Design review of the part shown in the three views and the two pictorial views. Dimensions are in mm from the part's minimum x, y and z. Round coordinates to 2 decimals unless told otherwise and drop trailing zeros. Write each loop counter-clockwise with the first axis right and the second up, starting at its lowest first coordinate (ties: lowest second). Pieces come first, ordered by that corner, then holes. Notation, with made-up numbers: (26.5, 32) - (56.5, 32) arc R30 ccw to (56.5, 71) - close; hole circle Ø1 at (18, 4.5). An arc over 180 degrees is marked (long way). Use one line per item in the form item = value.
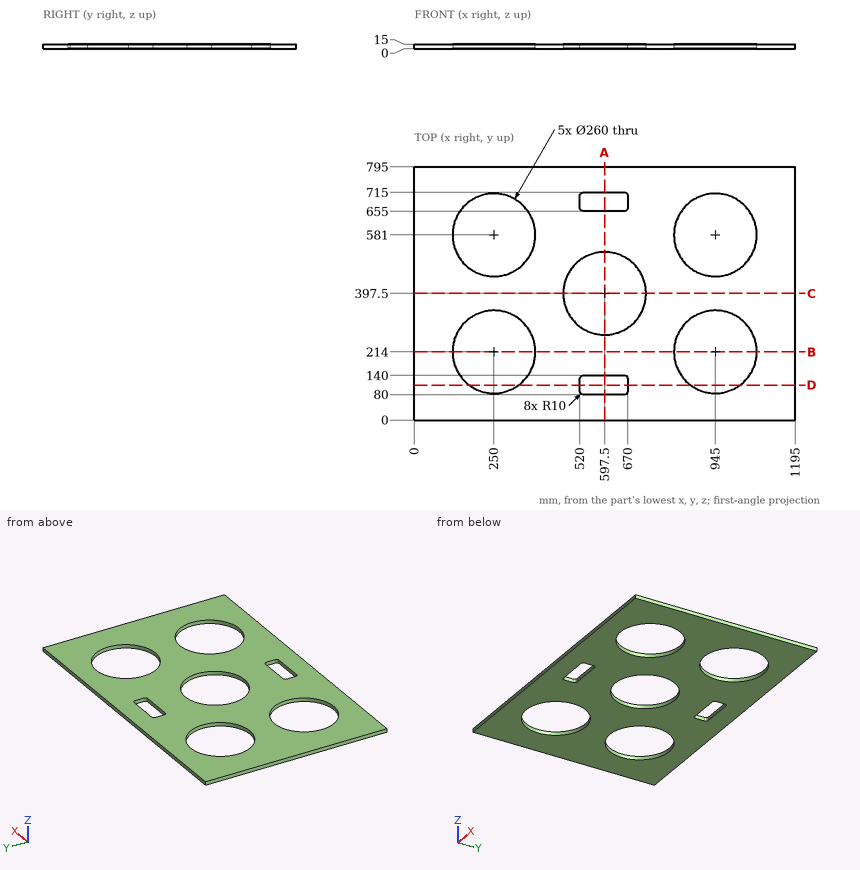
Q1. We need section D-D on y = 110. Write out the cut boundary in (x, z), then the cut area to 3 significant figures.
Calculated:
outline = (0, 0) - (172, 0) - (172, 15) - (0, 15) - close; (328, 0) - (520, 0) - (520, 15) - (328, 15) - close; (670, 0) - (867, 0) - (867, 15) - (670, 15) - close; (1023, 0) - (1195, 0) - (1195, 15) - (1023, 15) - close
area = 11,000 mm2
Q2. To check wall thickness, follow line 1 along Y through (x, z) = (945, 4.75); line 2 along X through (y, z) = (219.5, 2); line 3 along Y through (x, z) = (542.5, 11.5). State the ranges of each line that lie inside material, in increasing order. Write a range as from..to.
Calculated:
line_1 = 0..84, 344..451, 711..795
line_2 = 0..120.12, 379.88..815.12, 1074.88..1195
line_3 = 0..80, 140..279.71, 515.29..655, 715..795
Q3. We need section C-C on y = 397.5. Write out the cut boundary in (x, z).
Calculated:
outline = (0, 0) - (467.5, 0) - (467.5, 15) - (0, 15) - close; (727.5, 0) - (1195, 0) - (1195, 15) - (727.5, 15) - close
Q4. We need section A-A on x = 597.5. Write out the cut boundary in (y, z), then the cut area to 4 significant figures.
Calculated:
outline = (0, 0) - (80, 0) - (80, 15) - (0, 15) - close; (140, 0) - (267.5, 0) - (267.5, 15) - (140, 15) - close; (527.5, 0) - (655, 0) - (655, 15) - (527.5, 15) - close; (715, 0) - (795, 0) - (795, 15) - (715, 15) - close
area = 6,225 mm2
Q5. We need section B-B on y = 214. Write out the cut boundary in (x, z), then the cut area to 3 significant figures.
Calculated:
outline = (0, 0) - (120, 0) - (120, 15) - (0, 15) - close; (380, 0) - (815, 0) - (815, 15) - (380, 15) - close; (1075, 0) - (1195, 0) - (1195, 15) - (1075, 15) - close
area = 10,100 mm2
Q6. For P1, Ø5, axis at x = 539.5, y = 136.5, coming from the +Z side, flat-tipped, find the tip position at first contact; note if it passes through.
Calculated:
P1 = through
